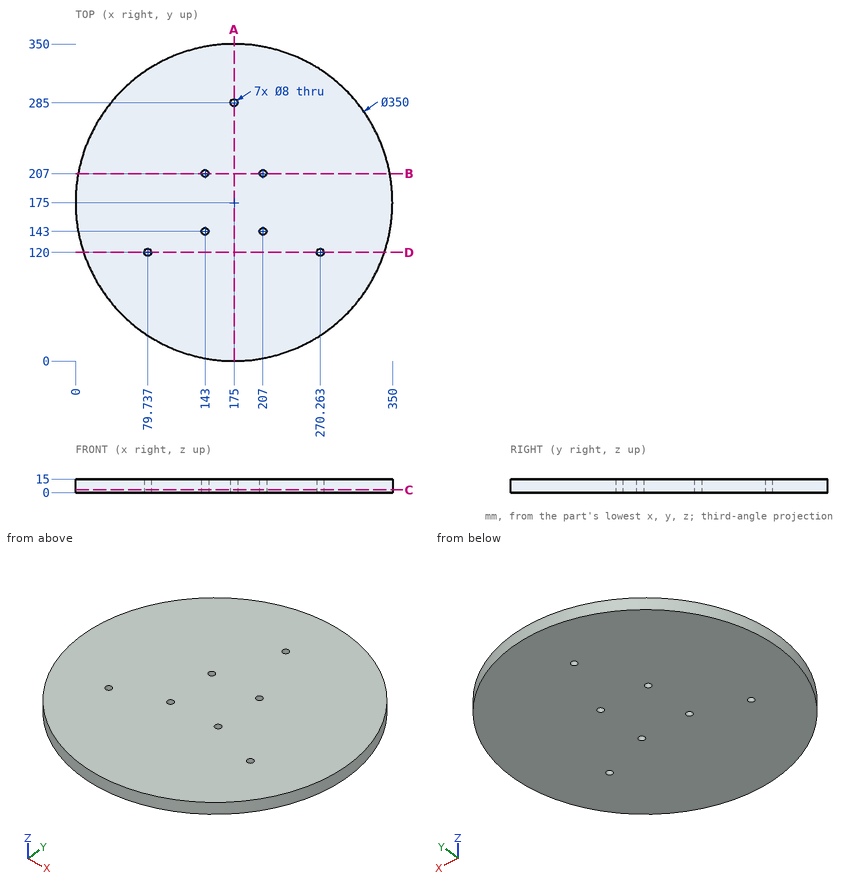
The drawing under review shows one solid part. Ordinate dimensions are in mm from its lowest x, y, z. Coordinates: 2 decimals unless noted, no trailing zeros. Write each loop counter-clockwise with the first axis right and the second up, starting at its lowest first coordinate (ties: lowest second). Pieces come first, ordered by that corner, then holes. Notation, with made-up numbers: (76.5, 58) - (98.5, 58) arc R12 ccw to (98.5, 65) - close; hole circle Ø3 at (-23.75, -1). An arc over 180 degrees is marked (long way). Answer in a Markdown table with one row per item. Add a question column.
Q1. We need section C-C, the plane z = 3. State the section outline as (x, y) points.
Q2. For P1, Ø10, axis at x = 262, y = 208, coming from the -Z side; P2, Ø2, axis at x = 185, z = 3, coming from the +Y side; P3, Ø1, axis at x = 75.5, z = 13, coming from the +Y side (1 decimal); P4, Ø8, axis at y = 243.5, z = 7, coming from the -X side, all flat-tipped, find the tip position at first contact; note any pin that passes through.
Q3. We need section A-A, the plane x = 175. State the section outline as (y, z) points.
Q4. We need section B-B, the plane y = 207. State the section outline as (x, z) points.
Q5. We need section D-D, the plane y = 120. State the section outline as (x, z) points, and give its area (3 significant figures).
Q6. For probe 1 along X at (y, z) = (121, 1.75); probe 2 along Y at (x, z) = (143, 3.5); probe 3 along X at (y, z) = (120, 11.5), list the stretches that pass through material, from the lowest coordinate up.
Answer list:
| question | item | result |
|---|---|---|
| 1 | outline | circle Ø350 at (175, 175); hole circle Ø8 at (79.74, 120); hole circle Ø8 at (143, 143); hole circle Ø8 at (143, 207); hole circle Ø8 at (175, 285); hole circle Ø8 at (207, 143); hole circle Ø8 at (207, 207); hole circle Ø8 at (270.26, 120) |
| 2 | P1 | stops at z = 0 |
| 2 | P2 | stops at y = 349.77 |
| 2 | P3 | stops at y = 319.3 |
| 2 | P4 | stops at x = 12.32 |
| 3 | outline | (0, 0) - (281, 0) - (281, 15) - (0, 15) - close; (289, 0) - (350, 0) - (350, 15) - (289, 15) - close |
| 4 | outline | (2.95, 0) - (139, 0) - (139, 15) - (2.95, 15) - close; (147, 0) - (203, 0) - (203, 15) - (147, 15) - close; (211, 0) - (347.05, 0) - (347.05, 15) - (211, 15) - close |
| 5 | outline | (8.87, 0) - (75.74, 0) - (75.74, 15) - (8.87, 15) - close; (83.74, 0) - (266.26, 0) - (266.26, 15) - (83.74, 15) - close; (274.26, 0) - (341.13, 0) - (341.13, 15) - (274.26, 15) - close |
| 5 | area | 4,740 mm2 |
| 6 | probe 1 | x = 8.54 to 75.86, 83.61 to 266.39, 274.14 to 341.46 |
| 6 | probe 2 | y = 2.95 to 139, 147 to 203, 211 to 347.05 |
| 6 | probe 3 | x = 8.87 to 75.74, 83.74 to 266.26, 274.26 to 341.13 |
